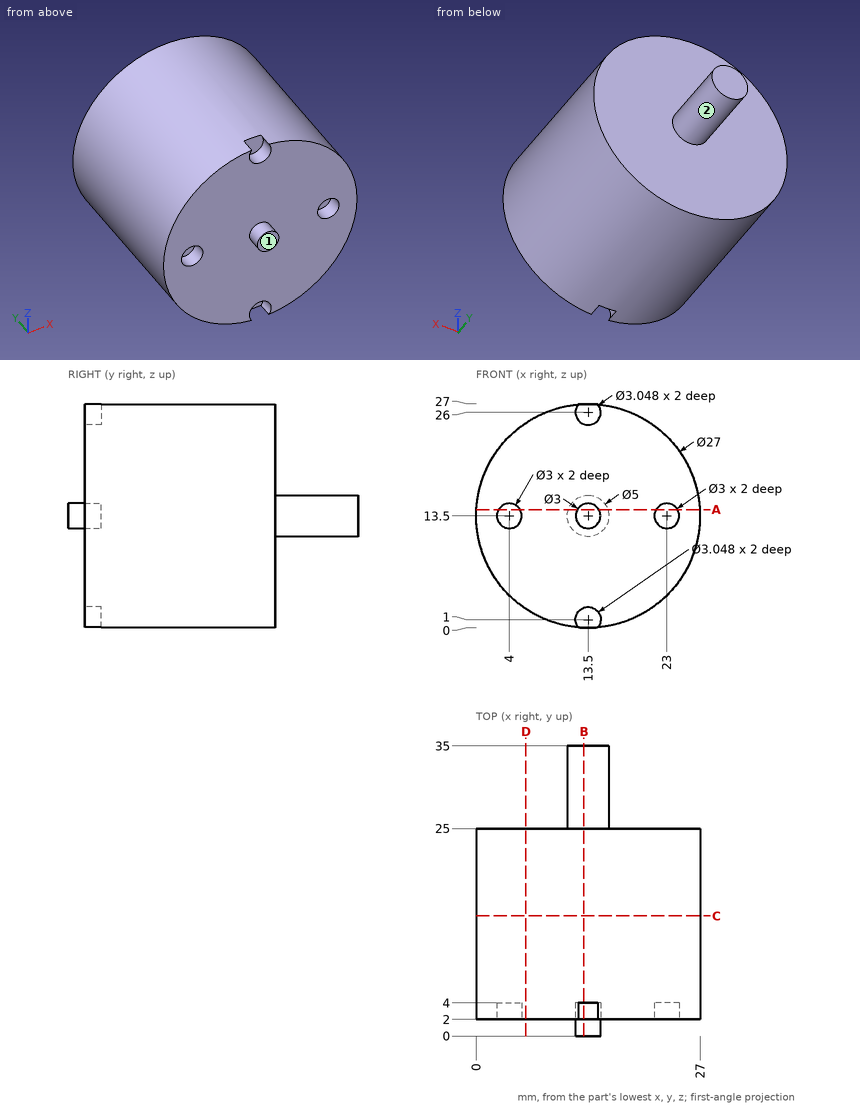
Verification items for this drawing (mm, ordinates from the low corner). A direction names the side the tool comes from. Coordinates: 2 decimals unless noted, no trailing zeros. Loops run counter-clockwise (first coordinate to the right, second up) from the corner with the lowest first, then second, coordinate; pieces in that order, holes last.
Item 1: Access from +Z, -Z, +X, -X, +Y, -Y to the whole of each face (thin tool, end or side, straight path). Record for the marked faces 1 and 2.
Item 2: Go/stop test with flat-tipped pins: pin 1 Ø12 at (x, z) = (4, 9) entering from -Y; pin 2 Ø3 at (y, z) = (10.5, 14.5) entering from -X; pin 3 Ø1 at (x, y) = (10.5, 13) entering from -Z; pin 4 Ø0.8 at (x, z) = (14, 26) entering from -Y. Record where each tip stops, or that it passes through.
Item 3: Sectioned sample at B-B, the plane x = 13. Record the boundary of the cut face in (y, z).
Item 4: Sectioned sample at C-C, the plane y = 14.5. Record the boundary of the cut face in (x, z), then the cut area to 3 significant figures.
Item 5: Sectioned sample at D-D, the plane x = 6. Record the boundary of the cut face in (y, z) (3 decimals).
Item 6: Sectioned sample at A-A, the plane z = 14.25. Record the boundary of the cut face in (x, y), then the cut area to 3 significant figures.
Item 7: Thickness scan on line 1 (Y direction, x = 16, z = 19.5); line 2 (Y direction, x = 15.25, z = 11.75); line 3 (X direction, y = 20.5, z = 23). Record the ranges inside material, lowest first.
Check result:
1. face 1: +Z, -Z, +X, -X, -Y
1. face 2: +Y
2. pin 1: stops at y = 2
2. pin 2: stops at x = 0
2. pin 3: stops at z = 0.23
2. pin 4: stops at y = 4
3. outline: (0, 12.09) - (2, 12.09) - (2, 2.44) - (4, 2.44) - (4, 0.01) - (25, 0.01) - (25, 11.05) - (35, 11.05) - (35, 15.95) - (25, 15.95) - (25, 26.99) - (4, 26.99) - (4, 24.56) - (2, 24.56) - (2, 14.91) - (0, 14.91) - close
4. outline: circle Ø27 at (13.5, 13.5)
4. area: 573 mm2
5. outline: (2, 2.275) - (25, 2.275) - (25, 24.725) - (2, 24.725) - close
6. outline: (0.02, 2) - (2.7, 2) - (2.7, 4) - (5.3, 4) - (5.3, 2) - (12.2, 2) - (12.2, 0) - (14.8, 0) - (14.8, 2) - (21.7, 2) - (21.7, 4) - (24.3, 4) - (24.3, 2) - (26.98, 2) - (26.98, 25) - (15.88, 25) - (15.88, 35) - (11.12, 35) - (11.12, 25) - (0.02, 25) - close
6. area: 663 mm2
7. line 1: y = 2 to 25
7. line 2: y = 2 to 35
7. line 3: x = 3.91 to 23.09
